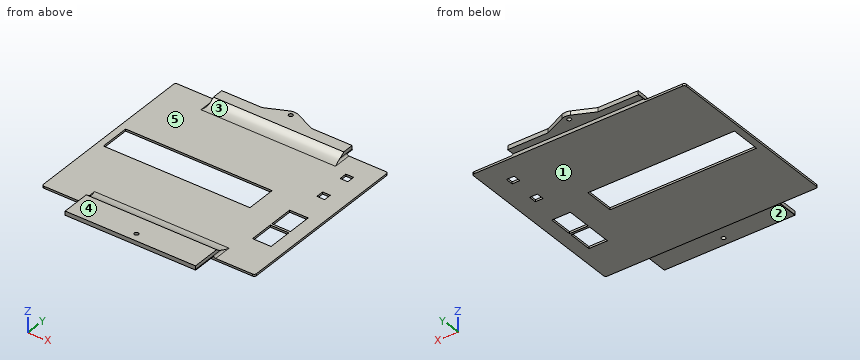
from build123d import *

# Parameters (mm, degrees)
SKETCH2_W           = 103.235
SKETCH2_H           = 87.36
SKETCH2_W_2         = 9
SKETCH2_H_2         = 11.625667
SKETCH2_W_3         = 3.751667
SKETCH2_H_3         = 3.751667
SKETCH2_W_4         = 71.061666
SKETCH2_H_4         = 14.546666
BOSS_EXTRUDE1_DEPTH = 1
BOSS_EXTRUDE2_START = -20
BOSS_EXTRUDE2_DEPTH = 63.235
FILLET1_R           = 10
FILLET2_R           = 1
FILLET4_R           = 1
BOSS_EXTRUDE3_DEPTH = 2
SKETCH5_R           = 1
CUT_EXTRUDE1_DEPTH  = 150.95559423


with BuildPart() as part:
    # Sketch2 → Boss-Extrude1 (new body)
    with BuildSketch(Plane.XY):
        with Locations((-77.235921563, -21.097735573)):
            Rectangle(SKETCH2_W, SKETCH2_H)
        with Locations((-36.618421563, -39.491569073)):
            Rectangle(SKETCH2_W_2, SKETCH2_H_2, mode=Mode.SUBTRACT)
        with Locations((-36.618421563, -26.791569073)):
            Rectangle(SKETCH2_W_2, SKETCH2_H_2, mode=Mode.SUBTRACT)
        with Locations((-36.299588063, -5.201569073)):
            Rectangle(SKETCH2_W_3, SKETCH2_H_3, mode=Mode.SUBTRACT)
        with Locations((-36.299588063, 10.038430927)):
            Rectangle(SKETCH2_W_3, SKETCH2_H_3, mode=Mode.SUBTRACT)
        with Locations((-90.105254563, -21.563402573)):
            Rectangle(SKETCH2_W_4, SKETCH2_H_4, mode=Mode.SUBTRACT)
    extrude(amount=BOSS_EXTRUDE1_DEPTH)

    # Sketch4 → Boss-Extrude2 (add)
    with BuildSketch(Plane.ZY.offset(128.853421563).offset(BOSS_EXTRUDE2_START)):
        Polygon((1.64, 23.082264427), (1.64, 26.082264427), (3.64, 26.082264427), (3.64, 20.582264427), (1, 20.582264427), (1, 22.582264427), (1.64, 22.582264427), align=None)
        Polygon((1.64, -76.617402573), (1.64, -73.617402573), (1.64, -64.777735573), (1, -64.777735573), (1, -62.777735573), (3.64, -62.777735573), (3.64, -76.617402573), align=None)
    extrude(amount=-BOSS_EXTRUDE2_DEPTH)

    # Fillet1
    # the kernel refuses this fillet: 10 mm, written as the material it adds along each edge
    with BuildSketch(Plane(origin=(-108.853421563, -62.777735573, 1), x_dir=(0, 1, 0), z_dir=(1, 0, 0))) as fillet1_piece_1:
        with BuildLine():
            CenterArc((6.769815359, 10), FILLET1_R, 227.39178247, 42.60821753)
            Line((0, 2.64), (-0.135396307, 2.4928))
            ThreePointArc((-0.135396307, 2.4928), (-0.2, 1.32), (-0.2, 0))
            Line((-0.2, 0), (0, -0.2))
            Line((0, -0.2), (6.769815359, -0.2))
            Line((6.769815359, -0.2), (6.769815359, 0))
        make_face()
    extrude(amount=63.235)
    with BuildSketch(Plane(origin=(-108.853421563, 20.582264427, 1), x_dir=(0, -1, 0), z_dir=(1, 0, 0))) as fillet1_piece_2:
        with BuildLine():
            CenterArc((6.769815359, -10), FILLET1_R, 90, 42.60821753)
            Line((0, -2.64), (-0.135396307, -2.4928))
            ThreePointArc((-0.135396307, -2.4928), (-0.2, -1.32), (-0.2, 0))
            Line((-0.2, 0), (0, 0.2))
            Line((0, 0.2), (6.769815359, 0.2))
            Line((6.769815359, 0.2), (6.769815359, 0))
        make_face()
    extrude(amount=63.235)

    # Fillet2
    fillet2_edges = [part.edges().sort_by_distance(p)[0] for p in [
        (-128.853421563, 22.582264427, 0.5),
        (-128.853421563, -64.777735573, 0.5),
        (-25.618421563, -64.777735573, 0.5),
        (-25.618421563, 22.582264427, 0.5),
    ]]
    fillet(fillet2_edges, radius=FILLET2_R)

    # Fillet4
    fillet4_edges = [part.edges().sort_by_distance(p)[0] for p in [
        (-45.618421563, -60.392827893, 1),
    ]]
    fillet(fillet4_edges, radius=FILLET4_R)
    fillet4_2_edges = [part.edges().sort_by_distance(p)[0] for p in [
        (-108.853421563, -60.392827893, 1),
    ]]
    fillet(fillet4_2_edges, radius=FILLET4_R)
    fillet4_3_edges = [part.edges().sort_by_distance(p)[0] for p in [
        (-45.618421563, 18.197356748, 1),
    ]]
    fillet(fillet4_3_edges, radius=FILLET4_R)
    fillet4_4_edges = [part.edges().sort_by_distance(p)[0] for p in [
        (-108.853421563, 18.197356748, 1),
    ]]
    fillet(fillet4_4_edges, radius=FILLET4_R)

    # Sketch6 → Boss-Extrude3 (add)
    with BuildSketch(Plane.XY.offset(3.64)):
        with BuildLine():
            Line((-89.306989375, 26.082264427), (-79.306989375, 30.633163033))
            ThreePointArc((-79.306989375, 30.633163033), (-77.235921563, 31.082264427), (-75.164853752, 30.633163033))
            Line((-75.164853752, 30.633163033), (-65.164853752, 26.082264427))
            Line((-65.164853752, 26.082264427), (-89.306989375, 26.082264427))
        make_face()
    extrude(amount=-BOSS_EXTRUDE3_DEPTH)

    # Sketch5 → Cut-Extrude1 (cut, through all)
    with BuildSketch(Plane.XY.offset(3.64)):
        with Locations((-77.235921563, -72.617402573)):
            Circle(SKETCH5_R)
        with Locations((-77.235921563, 28.582264427)):
            Circle(SKETCH5_R)
    extrude(amount=-CUT_EXTRUDE1_DEPTH, mode=Mode.SUBTRACT)


solid = part.part
Geometry: final body of the model. Coordinates: model frame, mm. Face numbers are marked on the shaded views. A direction names the side the tool comes from. Coordinates: 2 decimals unless noted, no trailing zeros. Loops run counter-clockwise (first coordinate to the right, second up) from the corner with the lowest first, then second, coordinate; pieces in that order, holes last. Notation, with made-up numbers: (-37.75, -22) - (-26.75, -22) arc R27 ccw to (-26.75, 4) - close; hole circle Ø8 at (-4.5, 32). An arc over 180 degrees is marked (long way). One line per question, with ' | ' between items. Start each with the question number.
(1) First-contact query: pin 1 (1.2 mm diameter, centred on x = -77.24, y = 28.58, fed in from +Z); pin 2 (3 mm diameter, centred on x = -60.5, y = -44.5, fed in from +Z); pin 3 (0.8 mm diameter, centred on x = -36, z = 0.5, fed in from -Y); pin 4 (0.8 mm diameter, centred on y = -66.5, z = 3, fed in from +X). Flat tips, straight axial feed; report the tip coordinate or a pass-through.
(2) Cut plane B-B on y = -26. Output: boundary loops of the cut face in (x, z).
(3) Reachability of the marked faces 1 and 2 from +Z, -Z, +X, -X, +Y, -Y: full face, straight path, thin tool, end or side. Return the list, or none.
(4) Cut plane D-D on x = -36. Output: boundary loops of the cut face in (y, z).
(5) Draft query along Y for the marked faces 3, 4 and 5. Return one class per face: +Y half, -Y half, draft (parallel to the pull), parting line (faces both ways), or undercut.
(6) Ray query, L1, parallel to X at y = -24.5, z = 0.2; L2, parallel to Y at x = -93.5, z = 2; L3, parallel to Y at x = -107, z = 0.9. Return the intervals inside material, ascending. Write a range as from..to.
(7) Cut plane C-C on z = 2.55. Output: boundary loops of the cut face in (x, y).
(8) Cut plane A-A on x = -119. Output: boundary loops of the cut face in (y, z), and give its area (3 significant figures).
Here are the results:
1) pin 1: through | pin 2: z = 1 | pin 3: y = -64.78 | pin 4: x = -45.62
2) outline: (-128.85, 0) - (-125.64, 0) - (-125.64, 1) - (-128.85, 1) - close; (-54.57, 0) - (-41.12, 0) - (-41.12, 1) - (-54.57, 1) - close; (-32.12, 0) - (-25.62, 0) - (-25.62, 1) - (-32.12, 1) - close
3) face 1: -Z, +X, -X, +Y, -Y | face 2: -Z, +X, -X, -Y
4) outline: (-64.78, 0) - (-45.3, 0) - (-45.3, 1) - (-64.78, 1) - close; (-33.68, 0) - (-32.6, 0) - (-32.6, 1) - (-33.68, 1) - close; (-20.98, 0) - (-7.08, 0) - (-7.08, 1) - (-20.98, 1) - close; (-3.33, 0) - (8.16, 0) - (8.16, 1) - (-3.33, 1) - close; (11.91, 0) - (22.58, 0) - (22.58, 1) - (11.91, 1) - close
5) face 3: undercut | face 4: draft | face 5: undercut
6) L1: -128.85..-125.64, -54.57..-41.12, -32.12..-25.62 | L2: -76.62..-60.37, 18.17..26.08 | L3: -64.78..-28.84, -14.29..22.58
7) outline: (-108.85, -76.62) - (-45.62, -76.62) - (-45.62, -61.36) - (-108.85, -61.36) - close; (-108.85, 19.16) - (-45.62, 19.16) - (-45.62, 26.08) - (-65.16, 26.08) - (-75.16, 30.63) arc R5 ccw to (-79.31, 30.63) - (-89.31, 26.08) - (-108.85, 26.08) - close; hole circle Ø2 at (-77.24, -72.62); hole circle Ø2 at (-77.24, 28.58)
8) outline: (-64.78, 0) - (-28.84, 0) - (-28.84, 1) - (-64.78, 1) - close; (-14.29, 0) - (22.58, 0) - (22.58, 1) - (-14.29, 1) - close | area: 72.8 mm²
